The drawing under review shows one solid part. Ordinate dimensions are in mm from its lowest x, y, z. Give positions to 0.01 mm unless a question says otherwise; leave off trailing zeros. Write each loop counter-clockwise with the first axis right and the second up, starting at its lowest first coordinate (ties: lowest second). Pieces come first, ordered by that corner, then holes.
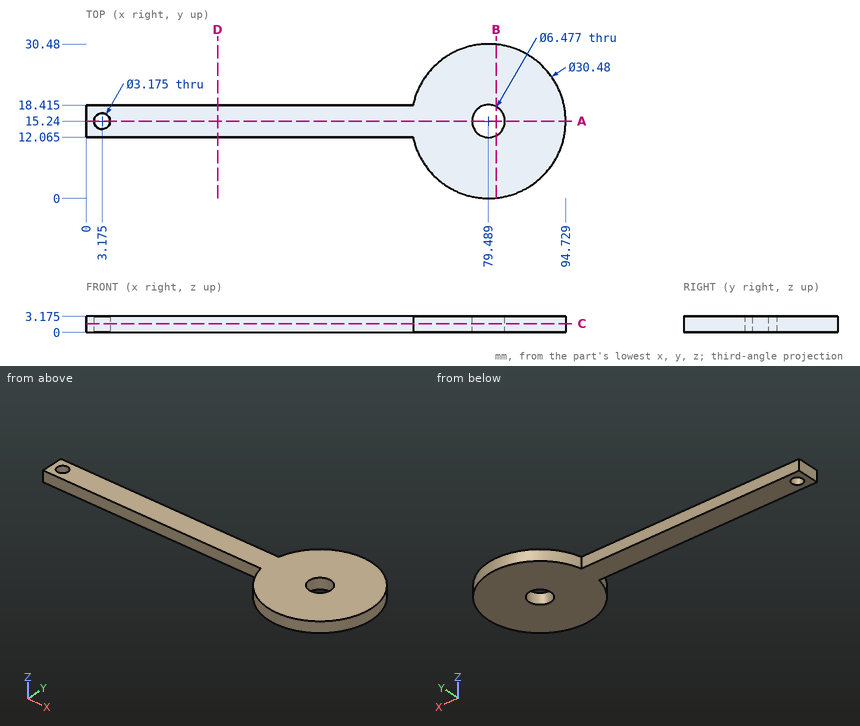
1) Consider section C-C, the plane z = 1.75. Give the boundary of the cut face in (x, y) (1 decimal).
2) Consider section A-A, the plane y = 15.24. Give the boundary of the cut face in (x, z) (1 decimal), then the cut area to 3 significant figures.
3) Insertion check: pin 1 (4 mm diameter, centred on x = 79.49, y = 15.24, fed in from +Z). The pin has a flat end and moves straight along its axis. Give the tip position at first contact, or say it passes through.
4) Consider section D-D, the plane x = 26. Give the boundary of the cut face in (y, z) (1 decimal).
5) Consider section B-B, the plane x = 81. Give the boundary of the cut face in (y, z) (1 decimal), then the cut area to 3 significant figures.
6) To check wall thickness, follow probe 1 along X at (y, z) = (15, 0.75) (1 decimal); probe 2 along X at (y, z) = (16, 2.3); probe 3 along Y at (x, z) = (38.5, 0.65) (1 decimal). State the ranges of each line that lie inside material, in increasing order.
Answer block:
1. outline: (0, 12.1) - (64.6, 12.1) arc R15.2 ccw (long way) to (64.6, 18.4) - (0, 18.4) - close; hole circle Ø3.2 at (3.2, 15.2); hole circle Ø6.5 at (79.5, 15.2)
2. outline: (0, 0) - (1.6, 0) - (1.6, 3.2) - (0, 3.2) - close; (4.8, 0) - (76.3, 0) - (76.3, 3.2) - (4.8, 3.2) - close; (82.7, 0) - (94.7, 0) - (94.7, 3.2) - (82.7, 3.2) - close
2. area: 270 mm2
3. pin 1: passes through
4. outline: (12.1, 0) - (18.4, 0) - (18.4, 3.2) - (12.1, 3.2) - close
5. outline: (0.1, 0) - (12.4, 0) - (12.4, 3.2) - (0.1, 3.2) - close; (18.1, 0) - (30.4, 0) - (30.4, 3.2) - (18.1, 3.2) - close
5. area: 78.1 mm2
6. probe 1: x = 0 to 1.6, 4.7 to 76.3, 82.7 to 94.7
6. probe 2: x = 0 to 1.78, 4.57 to 76.34, 82.64 to 94.71
6. probe 3: y = 12.1 to 18.4
